For this review, take the finished solid that the model builds, in its own axes (mm). Face numbers are marked on the shaded views. A direction names the side the tool comes from. Give positions to 0.01 mm unless a question says otherwise; leave off trailing zeros. Order: outer loops, then holes, each group sorted by start corner. A loop starts at its lowest first (then second) coordinate and runs counter-clockwise, first axis right, second up.
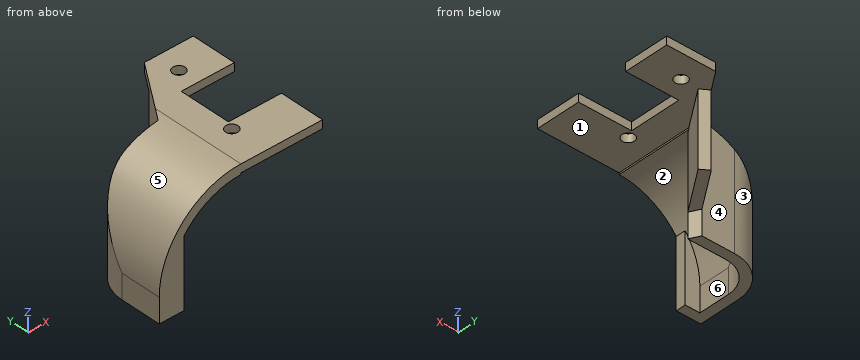
from build123d import *

# Parameters (mm, degrees)
F0_R      = 1.5
F1_DEPTH  = 2
F2_DEPTH  = 24
F4_DEPTH  = 25
F5_R      = 1.5
F6_DEPTH  = 24
F8_DEPTH  = 20
F10_DEPTH = 25
F11_DEPTH = 6


# Not quite as in the source:
# - a feature names something its author has since deleted; it is built from what else it names


with BuildPart() as f1:
    # F0 (on Top) → F1 (new body)
    with BuildSketch(Plane.XY):
        with BuildLine():
            Line((-20, -17.6375247538), (20, -17.6375247538))
            Line((20, -17.6375247538), (20, -6.6375247538))
            Line((20, -6.6375247538), (7, -6.6375247538))
            Line((7, -6.6375247538), (7, 6))
            Line((7, 6), (20, 6))
            Line((20, 6), (20, 17))
            Line((20, 17), (8, 17))
            Line((8, 17), (-2, 2.3624752462))
            Line((-2, 2.3624752462), (-10, 2.3624752462))
            ThreePointArc((-10, 2.3624752462), (-17.0710678119, -0.5664569419), (-20, -7.6375247538))
            Line((-20, -7.6375247538), (-20, -17.6375247538))
        make_face()
        with Locations((6, -8.6375247538)):
            Circle(F0_R, mode=Mode.SUBTRACT)
        with Locations((11, 11)):
            Circle(F0_R, mode=Mode.SUBTRACT)
    extrude(amount=F1_DEPTH)

    # F2 (add): a face of the model
    f2_faces = [f1.faces().sort_by_distance(p)[0] for p in [
        (0.9940051369, -4.5309976768, 0),
    ]]
    extrude(f2_faces, amount=F2_DEPTH)

    # F3 (on face) → F4 (cut)
    with BuildSketch(Plane.XZ.offset(17.6375247538)):
        with BuildLine():
            Line((-20, -11), (-20, -18))
            ThreePointArc((-20, -18), (-14.1421356237, -3.8578643763), (0, 2))
            Line((0, 2), (-7, 2))
            Line((-7, 2), (-20, 2))
            Line((-20, 2), (-20, -11))
        make_face()
    extrude(amount=-F4_DEPTH, mode=Mode.SUBTRACT)

    # F5 (on face) → F6 (cut)
    with BuildSketch(Plane(origin=(0, 0, -24), x_dir=(1, 0, 0), z_dir=(0, 0, -1))):
        with BuildLine():
            Line((20, 17.6375247538), (-14, 17.6375247538))
            Line((-14, 17.6375247538), (-14, 15.2375247538))
            Line((-14, 15.2375247538), (-17.6, 15.2375247538))
            Line((-17.6, 15.2375247538), (-17.6, 7.6375247538))
            ThreePointArc((-17.6, 7.6375247538), (-15.374011537, 2.2635132168), (-10, 0.0375247538))
            Line((-10, 0.0375247538), (-0.7330154527, 0.0375247538))
            Line((-0.7330154527, 0.0375247538), (6.7509134438, -10.9170946941))
            Line((6.7509134438, -10.9170946941), (4.7692207252, -12.2709388392))
            Line((4.7692207252, -12.2709388392), (8, -17))
            Line((8, -17), (20, -17))
            Line((20, -17), (20, -6))
            Line((20, -6), (7, -6))
            Line((7, -6), (7, 6.6375247538))
            Line((7, 6.6375247538), (20, 6.6375247538))
            Line((20, 6.6375247538), (20, 17.6375247538))
        make_face()
        with Locations((11, -11)):
            Circle(F5_R, mode=Mode.SUBTRACT)
        with Locations((6, 8.6375247538)):
            Circle(F5_R, mode=Mode.SUBTRACT)
    extrude(amount=-F6_DEPTH, mode=Mode.SUBTRACT)

    # F7 (on face) → F8 (join)
    with BuildSketch(Plane.XZ.offset(17.6375247538)):
        with BuildLine():
            Line((0, -0.4), (0, 2))
            ThreePointArc((0, 2), (-14.1421356237, -3.8578643763), (-20, -18))
            Line((-20, -18), (-17.6, -18))
            ThreePointArc((-17.6, -18), (-12.4450793489, -5.5549206511), (0, -0.4))
        make_face()
    extrude(amount=-F8_DEPTH)

    # F9 (on face) → F10 (cut)
    with BuildSketch(Plane(origin=(0, 0, -24), x_dir=(1, 0, 0), z_dir=(0, 0, -1))):
        with BuildLine():
            ThreePointArc((-25, 7.6375247538), (-20.6066017178, -2.969076964), (-10, -7.3624752462))
            Line((-10, -7.3624752462), (-10, -2.3624752462))
            ThreePointArc((-10, -2.3624752462), (-17.0710678119, 0.5664569419), (-20, 7.6375247538))
            Line((-20, 7.6375247538), (-25, 7.6375247538))
        make_face()
    extrude(amount=-F10_DEPTH, mode=Mode.SUBTRACT)

    # F5 (on face) → F11 (cut)
    with BuildSketch(Plane(origin=(0, 0, -24), x_dir=(1, 0, 0), z_dir=(0, 0, -1))):
        Polygon((-0.7330154527, 0.0375247538), (-2, -2.3624752462), (4.7692207252, -12.2709388392), (6.7509134438, -10.9170946941), align=None)
    extrude(amount=-F11_DEPTH, mode=Mode.SUBTRACT)


solid = f1.part
1) We need section B-B on x = 6. Give the boundary of the cut face in (y, z).
Answer sheet:
outline: (-17.64, 0) - (-10.14, 0) - (-10.14, 2) - (-17.64, 2) - close; (-7.14, 0) - (9.82, 0) - (9.82, -18) - (11.43, -18) - (11.43, 0) - (14.07, 0) - (14.07, 2) - (-7.14, 2) - close
2) We need section D-D on z = -4.5. Give the boundary of the cut face in (x, y), then the cut area to 3 significant figures.
Answer sheet:
outline: (-14.76, -17.64) - (-11.29, -17.64) - (-11.29, -0.15) arc R7.6 cw to (-10, -0.04) - (-0.73, -0.04) - (6.75, 10.92) - (4.77, 12.27) - (-2, 2.36) - (-10, 2.36) arc R10 ccw to (-14.76, 1.16) - close
area: 122 mm2
3) Draft analysis for pull direction Y (two halves, no side actions). For the marked faces 1, 2 and 3, state which applies: +Y half, -Y half, draft (parallel to the pull), parting line (faces both ways), or undercut.
Answer sheet:
face 1: draft
face 2: undercut
face 3: +Y half
4) We need section C-C on y = -13. Give the boundary of the cut face in (x, z).
Answer sheet:
outline: (-20, -24) - (-17.6, -24) - (-17.6, -18) arc R17.6 cw to (0, -0.4) - (0, 0) - (20, 0) - (20, 2) - (0, 2) arc R20 ccw to (-20, -18) - close
5) Clearance check with flat-ended pins moving along their axes: pin 1 (5 mm diameter, centred on y = -6, z = -12.5, fed in from -X); pin 2 (6 mm diameter, centred on x = 0, y = -4.5, fed in from -Z); pin 3 (1.2 mm diameter, centred on y = -16.5, z = -18.5, fed in from +X); pin 4 (2.5 mm diameter, centred on x = 6, y = -8.64, fed in from -Z). State where each tip first meets the part, or that it passes through.
Answer sheet:
pin 1: stops at x = -19.77
pin 2: stops at z = -0.66
pin 3: stops at x = -14
pin 4: passes through
6) To check wall thickness, follow line 1 (Y direction, x = 11, z = 0.7); line 2 (Y direction, x = 6, z = 1.1); line 3 (Z direction, x = 6, y = -5). State the ranges of each line that lie inside material, in increasing order.
Answer sheet:
line 1: y = -17.64 to -6.64, 6 to 9.5, 12.5 to 17
line 2: y = -17.64 to -10.14, -7.14 to 14.07
line 3: z = 0 to 2
7) We need section A-A on x = 11. Give the boundary of the cut face in (y, z).
Answer sheet:
outline: (-17.64, 0) - (-6.64, 0) - (-6.64, 2) - (-17.64, 2) - close; (6, 0) - (9.5, 0) - (9.5, 2) - (6, 2) - close; (12.5, 0) - (17, 0) - (17, 2) - (12.5, 2) - close
8) Tool access review of the marked faces 4, 5 and 6: name each direction out of +Z, -Z, +X, -X, +Y, -Y from which nothing blocks a thin tool from reaching the whole face with its end or side.
Answer sheet:
face 4: +Z, -Z, -X, +Y
face 5: +Z, -X, +Y, -Y
face 6: -Z, +X
